Check sheet for the modelled part. Datum: model origin and axes. Units: mm. A direction names the side the tool comes from. Give positions to 0.01 mm unless a question says otherwise; leave off trailing zeros. Write each loop counter-clockwise with the first axis right and the second up, starting at its lowest first coordinate (ties: lowest second). Pieces come first, ordered by that corner, then holes. Notation, with made-up numbers: (0.25, -9) -> (39.25, -9) arc R11 cw to (39.25, 10) -> close; hole circle Ø9 at (7.25, 38). An arc over 180 degrees is marked (long way). Use a Markdown table: item, result. Add a question column.
1. Cross-section at C-C (z = 34.5). Enter the section's corners in (x, y).
2. Cross-section at B-B (y = -15.75). Enter the section's corners in (x, z).
3. Set-up check for faces 5 (the cylindrical face through (-22.7, -18.71, 15.76)), 6 (the flat face through (-30.934, -8, 41)), 7 (the cylindrical face through (-39.166, -0.285, 30.162)): record each of +Z, -Z, +X, -X, +Y, -Y from which the full face is reachable in a straight line by a thin tool's end or side.
4. Cross-section at A-A (z = 19). Enter the section's corners in (x, y).
5. Scan lines: probe 1 along X at (y, z) = (-3, 19.5); probe 2 along Z at (x, y) = (-23, -17.25); probe 3 along Y at (x, z) = (-34, 21.5). Record each from-to range of solid material in increasing order. Write a range as [from, to].
6. Release check for a two-part mould opening along X. For faces 1 (the flat face through (-35, -16.5, 24)), 2 (the flat face through (-40.434, -9, 23)), 3 (the flat face through (-35, -8, 17.962)), 4 (the flat face through (-31, 0, 27)) record: released by +X, released by -X, zero draft, split by the parting line, or undercut.
7. Gauge pin test, flat ends, axial feed: P1, Ø8, axis at y = -6.5, z = 38.5, coming from the +X side; P2, Ø3, axis at x = -28, y = -12, coming from the -Z side; P3, Ø2.5, axis at x = -35, z = 24, coming from the +Y side. Record the tip position at first contact, or that the pin passes through.
8. Cross-section at D-D (x = -25.5). Enter the section's corners in (y, z), then the cut area to 3 significant figures.
from build123d import *

# Parameters (mm, degrees)
F0_W     = 10
F0_H     = 15
F1_DEPTH = 19
F2_T     = -2.5
F3_DEPTH = 9
F4_T     = -2.5
F5_DEPTH = 25
F6_DEPTH = 25
F8_DEPTH = 22
F9_R     = 1


# Not quite as in the source:
# - two fillets or chamfers of one size are made in one step


with BuildPart() as f1:
    # F0 (on Front) → F1 (new body)
    with BuildSketch(Plane.XZ):
        with Locations((-35.433777729, 22.9624143615)):
            Rectangle(F0_W, F0_H)
    extrude(amount=F1_DEPTH)

    # F2
    f2_openings = [f1.faces().sort_by_distance(p)[0] for p in [
        (-35.433778, 0, 22.962414),
        (-35.433778, -9.5, 30.462414),
    ]]
    offset(amount=F2_T, openings=f2_openings)

    # F3 (add): a face of the model
    f3_faces = [f1.faces().sort_by_distance(p)[0] for p in [
        (-30.433777729, -9.5, 22.9624143615),
    ]]
    extrude(f3_faces, amount=F3_DEPTH)

    # F4: a shell. OpenCascade refuses it in one call, so the cavity is built on its own and cut out:
    # the body offset inwards by the wall thickness, plus a prism from it out through each open face.
    f4_core = offset(f1.part, amount=F4_T, kind=Kind.INTERSECTION, mode=Mode.PRIVATE)
    f4_exits = [f4_core.faces().sort_by_distance(p)[0] for p in [
        (-27.183778, -2.5, 22.962414),
    ]]
    add(f4_core, mode=Mode.SUBTRACT)
    extrude(f4_exits, amount=-F4_T, mode=Mode.SUBTRACT)

    # F5 (cut): a face of the model
    f5_faces = [f1.faces().sort_by_distance(p)[0] for p in [
        (-27.183777729, -16.5, 22.9624143615),
    ]]
    extrude(f5_faces, amount=-F5_DEPTH, mode=Mode.SUBTRACT)

    # F6 (cut): a face of the model
    f6_faces = [f1.faces().sort_by_distance(p)[0] for p in [
        (-27.183777729, -9.5, 17.9624143615),
    ]]
    extrude(f6_faces, amount=-F6_DEPTH, mode=Mode.SUBTRACT)

    # F7 (on face) → F8 (join)
    with BuildSketch(Plane.XY.offset(30.4624143615)):
        Polygon((-30.933777729, 0), (-32.933777729, 0), (-32.933777729, -17.8228756555), (-31.933777729, -17.8228756555), (-31.433777729, -17.8228756555), (-30.433777729, -16.5), (-30.933777729, -16.5), align=None)
    extrude(amount=F8_DEPTH)

    # F9
    f9_edges = [f1.edges().sort_by_distance(p)[0] for p in [
        (-22.683778, 0, 15.462414),
        (-22.683778, -19, 15.462414),
        (-39.183778, 0, 30.462414),
    ]]
    fillet(f9_edges, radius=F9_R)


solid = f1.part
Worked answers:
| question | item | result |
|---|---|---|
| 1 | outline | (-32.93, -17.82) -> (-31.43, -17.82) -> (-30.43, -16.5) -> (-30.93, -16.5) -> (-30.93, 0) -> (-32.93, 0) -> close |
| 2 | outline | (-40.43, 15.46) -> (-30.43, 15.46) -> (-30.43, 27.96) -> (-23.93, 27.96) -> (-23.93, 15.46) -> (-21.43, 15.46) -> (-21.43, 30.46) -> (-30.93, 30.46) -> (-30.93, 52.46) -> (-32.93, 52.46) -> (-32.93, 17.96) -> (-37.93, 17.96) -> (-37.93, 30.46) -> (-40.43, 30.46) -> close |
| 3 | face 5 | -Z, +X, -Y |
| 3 | face 6 | +Z, +X, +Y |
| 3 | face 7 | +Z, -X, +Y |
| 4 | outline | (-40.43, -19) -> (-30.43, -19) -> (-30.43, 0) -> (-32.93, 0) -> (-32.93, -16.5) -> (-37.93, -16.5) -> (-37.93, 0) -> (-40.43, 0) -> close; (-23.93, -19) -> (-21.43, -19) -> (-21.43, 0) -> (-23.93, 0) -> close |
| 5 | probe 1 | x = [-40.43, -37.93], [-32.93, -30.43], [-23.93, -21.43] |
| 5 | probe 2 | z = [15.46, 30.46] |
| 5 | probe 3 | y = [-19, -16.5] |
| 6 | face 1 | undercut |
| 6 | face 2 | released by -X |
| 6 | face 3 | undercut |
| 6 | face 4 | zero draft |
| 7 | P1 | stops at x = -30.93 |
| 7 | P2 | stops at z = 27.96 |
| 7 | P3 | stops at y = -16.5 |
| 8 | outline | (-19, 27.96) -> (0, 27.96) -> (0, 30.46) -> (-19, 30.46) -> close |
| 8 | area | 47.5 mm² |
